```python
from build123d import *

# Parameters (mm, degrees)
SKETCH1_W           = 27.2
SKETCH1_H           = 23.9
BOSS_EXTRUDE1_DEPTH = 30
SHELL1_T            = -3.5
BOSS_EXTRUDE2_DEPTH = 13.7
SHELL3_START        = -10.2
SHELL3_DEPTH        = 20.4
FILLET2_R           = 2
SKETCH3_R           = 2.1
CUT_EXTRUDE1_DEPTH  = 97.890637096
FILLET3_R           = 10


# Read off the part's stored shape, not the designer's step: Shell3
with BuildPart() as part:
    # Sketch1 → Boss-Extrude1 (new, symmetric)
    with BuildSketch(Plane(origin=(0, 0, 0), x_dir=(0, 0, -1), z_dir=(1, 0, 0))):
        Rectangle(SKETCH1_W, SKETCH1_H)
    extrude(amount=BOSS_EXTRUDE1_DEPTH, both=True)

    # Shell1
    shell1_openings = [part.faces().sort_by_distance(p)[0] for p in [
        (30, 0, 0),
        (-30, 0, 0),
        (0, 11.95, 0),
    ]]
    offset(amount=SHELL1_T, openings=shell1_openings, kind=Kind.INTERSECTION)

    # Sketch2 → Boss-Extrude2 (add, symmetric)
    with BuildSketch(Plane(origin=(0, 0, 0), x_dir=(0, 0, -1), z_dir=(1, 0, 0))):
        Polygon((0.263208782, -11.95), (32.763208782, -68.241651246), (53.114805771, -56.491651246), (13.6, 11.95), (13.6, -11.95), align=None)
    extrude(amount=BOSS_EXTRUDE2_DEPTH, both=True)

    # Shell3 outline → Shell3 (cut)
    with BuildSketch(Plane.YZ.offset(SHELL3_START)):
        Polygon((8.45, -15.620725942), (8.45, -13.6), (-11.95, -13.6), (-11.95, -4.304660666), (-66.491651246, -35.794297695), (-56.491651246, -53.114805771), align=None)
    extrude(amount=SHELL3_DEPTH, mode=Mode.SUBTRACT)

    # Fillet2
    fillet2_edges = [part.edges().sort_by_distance(p)[0] for p in [
        (0, -11.95, 13.6),
    ]]
    fillet(fillet2_edges, radius=FILLET2_R)

    # Sketch3 → Cut-Extrude1 (cut, through all)
    with BuildSketch(Plane(origin=(13.7, 0, 0), x_dir=(0, 0, -1), z_dir=(1, 0, 0))):
        with Locations((40.954551733, -55.429473419)):
            Circle(SKETCH3_R)
        with Locations((30.954551733, -38.108965344)):
            Circle(SKETCH3_R)
        with Locations((20.954551733, -20.788457268)):
            Circle(SKETCH3_R)
    extrude(amount=-CUT_EXTRUDE1_DEPTH, mode=Mode.SUBTRACT)

    # Fillet3
    fillet3_edges = [part.edges().sort_by_distance(p)[0] for p in [
        (0, -11.95, -0.263208782),
    ]]
    fillet(fillet3_edges, radius=FILLET3_R)


solid = part.part
```
Work out the finished part from the listing and answer in its coordinate system (mm). A direction names the side the tool comes from. Give positions to 0.01 mm unless a question says otherwise; leave off trailing zeros. Loops run counter-clockwise (first coordinate to the right, second up) from the corner with the lowest first, then second, coordinate; pieces in that order, holes last. Notation, with made-up numbers: (44.5, 25.25) -> (64.5, 25.25) arc R17 cw to (64.5, 55.25) -> close; hole circle Ø5 at (20.25, 11.5). An arc over 180 degrees is marked (long way). Put each result on its own line as item: value. Start each with the question number.
Item 1: Each of these flat-tipped pins is pushed along its axis until it touches: P1, Ø8, axis at y = -16, z = -4.5, coming from the -X side; P2, Ø7.5, axis at x = 1, z = -7.5, coming from the -Y side; P3, Ø1, axis at x = 18, z = -9.5, coming from the +Y side; P4, Ø10, axis at x = 19.5, y = -25.5, coming from the +Z side. Where does it stop, or does it pass through?
Item 2: Which of the six approach directions +Z, -Z, +X, -X, +Y, -Y give full straight-line access (tool end or side, diameter ignored) to faces 1 (the face through (0, 2, 10.1)), 2 (the face through (22, 0, -13.6)), 3 (the face through (0, -11.95, 8)), 4 (the face through (-0.14, -38.84, -19.83))?
Item 3: The part is cut by section A-A (z = -48). Give the vertices of the cut face in (x, y), then the cut area to 3 significant figures.
Item 4: The part is cut by section C-C (x = -2). Give the vertices of the cut face in (y, z).
Item 5: The part is cut by section D-D (z = -30.5). Give the vertices of the cut face in (x, y).
Item 6: The part is cut by section B-B (y = 2). Give the vertices of the cut face in (x, z), then the cut area to 3 significant figures.
Item 7: The mould has two halves that part along X. Classify faces 5 (the face through (0, -11.95, -9)), 6 (the face through (30, -9, 2)), 7 (the face through (0, -8.45, 0)): released by +X, released by -X, zero draft, split by the parting line, or undercut.
Item 8: Find the intervals of material crossed by L1, parallel to Z at x = 21.5, y = 5; L2, parallel to X at y = -18.5, z = -30.5; L3, parallel to Y at x = 1, z = -5, in increasing order. Write a range as [from, to].
Answers below:
1. P1: x = -13.7
1. P2: y = -30.98
1. P3: y = -8.45
1. P4: through
2. face 1: +X, -X, +Y
2. face 2: -Z, +X, +Y, -Y
2. face 3: +Z, -Y
2. face 4: -Z
3. outline: (-13.7, -59.44) -> (-10.2, -59.44) -> (-10.2, -47.63) -> (-13.7, -47.63) -> close; (10.2, -59.44) -> (13.7, -59.44) -> (13.7, -47.63) -> (10.2, -47.63) -> close
3. area: 82.7 mm2
4. outline: (-68.24, -32.76) -> (-66.49, -35.79) -> (-11.95, -4.3) -> (-11.95, -13.6) -> (8.45, -13.6) -> (8.45, -15.62) -> (11.95, -13.6) -> (11.95, -10.1) -> (-8.45, -10.1) -> (-8.45, 10.1) -> (11.95, 10.1) -> (11.95, 13.6) -> (-9.95, 13.6) arc R2 ccw to (-11.95, 11.6) -> (-11.95, 5.51) arc R10 cw to (-16.95, -3.15) -> close
5. outline: (-13.7, -64.32) -> (13.7, -64.32) -> (13.7, -40.16) -> (10.2, -40.16) -> (10.2, -57.32) -> (-10.2, -57.32) -> (-10.2, -40.16) -> (-13.7, -40.16) -> close; (-13.7, -36.06) -> (-10.2, -36.06) -> (-10.2, -17.32) -> (-13.7, -17.32) -> close; (10.2, -36.06) -> (13.7, -36.06) -> (13.7, -17.32) -> (10.2, -17.32) -> close
6. outline: (-30, -13.6) -> (-13.7, -13.6) -> (-13.7, -19.34) -> (-10.2, -19.34) -> (-10.2, -13.6) -> (10.2, -13.6) -> (10.2, -19.34) -> (13.7, -19.34) -> (13.7, -13.6) -> (30, -13.6) -> (30, -10.1) -> (-30, -10.1) -> close; (-30, 10.1) -> (30, 10.1) -> (30, 13.6) -> (-30, 13.6) -> close
6. area: 460 mm2
7. face 5: undercut
7. face 6: released by +X
7. face 7: zero draft
8. L1: [-13.6, -10.1], [10.1, 13.6]
8. L2: [-13.7, -10.2], [10.2, 13.7]
8. L3: [-20.15, -13.15], [-11.95, -8.45]
